```python
from build123d import *

# Parameters (mm, degrees)
F1_W     = 3
F1_H     = 5.5
F1_H_2   = 7.5
F1_H_3   = 5
F1_H_4   = 3
F1_W_2   = 17.5
F1_W_3   = 10
F2_DEPTH = 3
F3_DEPTH = 20
F0_W     = 5
F0_H     = 5
F0_R     = 1.5
F4_DEPTH = 11
F5_DEPTH = 15
F6_R     = 2
F1_H_5   = 59
F7_DEPTH = 1


with BuildPart() as f2:
    # F1 (on Top) → F2 (new body)
    with BuildSketch(Plane.XY):
        with Locations((-6.5, -41.25)):
            Rectangle(F1_W, F1_H)
        with Locations((-6.5, 40.25)):
            Rectangle(F1_W, F1_H_2)
        with Locations((-6.5, 34)):
            Rectangle(F1_W, F1_H_3)
        with Locations((-6.5, 30)):
            Rectangle(F1_W, F1_H_4)
        with Locations((-6.5, -36)):
            Rectangle(F1_W, F1_H_3)
        with Locations((-6.5, -32)):
            Rectangle(F1_W, F1_H_4)
        Polygon((43, -47), (43, -44), (25.5, -44), (8, -44), (5, -44), (-5, -44), (-8, -44), (-25.5, -44), (-43, -44), (-43, -47), align=None)
        Polygon((43, -38.5), (43, -44), (43, -47), (46, -47), (46, 47), (-46, 47), (-46, -47), (-43, -47), (-43, -44), (-43, -38.5), (-43, -33.5), (-43, -30.5), (-43, 28.5), (-43, 31.5), (-43, 36.5), (-43, 44), (-25.5, 44), (-8, 44), (-5, 44), (5, 44), (8, 44), (25.5, 44), (43, 44), (43, 36.5), (43, 31.5), (43, 28.5), (43, -30.5), (43, -33.5), align=None)
        with Locations((-34.25, 40.25)):
            Rectangle(F1_W_2, F1_H_2)
        with Locations((0, 40.25)):
            Rectangle(F1_W_3, F1_H_2)
        with Locations((6.5, 40.25)):
            Rectangle(F1_W, F1_H_2)
        with Locations((34.25, 40.25)):
            Rectangle(F1_W_2, F1_H_2)
        with Locations((34.25, 34)):
            Rectangle(F1_W_2, F1_H_3)
        with Locations((6.5, 34)):
            Rectangle(F1_W, F1_H_3)
        with Locations((-34.25, 34)):
            Rectangle(F1_W_2, F1_H_3)
        with Locations((0, 34)):
            Rectangle(F1_W_3, F1_H_3)
        with Locations((-34.25, 30)):
            Rectangle(F1_W_2, F1_H_4)
        with Locations((6.5, 30)):
            Rectangle(F1_W, F1_H_4)
        with Locations((34.25, 30)):
            Rectangle(F1_W_2, F1_H_4)
        with Locations((0, 30)):
            Rectangle(F1_W_3, F1_H_4)
        with Locations((0, -41.25)):
            Rectangle(F1_W_3, F1_H)
        with Locations((0, -36)):
            Rectangle(F1_W_3, F1_H_3)
        with Locations((0, -32)):
            Rectangle(F1_W_3, F1_H_4)
        with Locations((6.5, -41.25)):
            Rectangle(F1_W, F1_H)
        with Locations((6.5, -36)):
            Rectangle(F1_W, F1_H_3)
        with Locations((6.5, -32)):
            Rectangle(F1_W, F1_H_4)
        with Locations((-34.25, -32)):
            Rectangle(F1_W_2, F1_H_4)
        with Locations((34.25, -32)):
            Rectangle(F1_W_2, F1_H_4)
        with Locations((34.25, -36)):
            Rectangle(F1_W_2, F1_H_3)
        with Locations((-34.25, -36)):
            Rectangle(F1_W_2, F1_H_3)
        with Locations((-34.25, -41.25)):
            Rectangle(F1_W_2, F1_H)
        with Locations((34.25, -41.25)):
            Rectangle(F1_W_2, F1_H)
    extrude(amount=F2_DEPTH)

    # F1 (on Top) → F3 (join)
    with BuildSketch(Plane.XY):
        Polygon((43, -38.5), (43, -44), (43, -47), (46, -47), (46, 47), (-46, 47), (-46, -47), (-43, -47), (-43, -44), (-43, -38.5), (-43, -33.5), (-43, -30.5), (-43, 28.5), (-43, 31.5), (-43, 36.5), (-43, 44), (-25.5, 44), (-8, 44), (-5, 44), (5, 44), (8, 44), (25.5, 44), (43, 44), (43, 36.5), (43, 31.5), (43, 28.5), (43, -30.5), (43, -33.5), align=None)
    extrude(amount=F3_DEPTH)

    # F0 (on Top) → F4 (join)
    with BuildSketch(Plane.XY):
        with Locations((37.5, 34)):
            Rectangle(F0_W, F0_H)
        with Locations((37.5, 34)):
            Circle(F0_R, mode=Mode.SUBTRACT)
        with Locations((2.5, 34)):
            Rectangle(F0_W, F0_H)
        with Locations((2.5, 34)):
            Circle(F0_R, mode=Mode.SUBTRACT)
        with Locations((-2.5, 34)):
            Rectangle(F0_W, F0_H)
        with Locations((-2.5, 34)):
            Circle(F0_R, mode=Mode.SUBTRACT)
        with Locations((-37.5, 34)):
            Rectangle(F0_W, F0_H)
        with Locations((-37.5, 34)):
            Circle(F0_R, mode=Mode.SUBTRACT)
        with Locations((37.5, -36)):
            Rectangle(F0_W, F0_H)
        with Locations((37.5, -36)):
            Circle(F0_R, mode=Mode.SUBTRACT)
        with Locations((-2.5, -36)):
            Rectangle(F0_W, F0_H)
        with Locations((-2.5, -36)):
            Circle(F0_R, mode=Mode.SUBTRACT)
        with Locations((2.5, -36)):
            Rectangle(F0_W, F0_H)
        with Locations((2.5, -36)):
            Circle(F0_R, mode=Mode.SUBTRACT)
        with Locations((-37.5, -36)):
            Rectangle(F0_W, F0_H)
        with Locations((-37.5, -36)):
            Circle(F0_R, mode=Mode.SUBTRACT)
        with Locations((37.5, 34)):
            Circle(F0_R)
        with Locations((2.5, 34)):
            Circle(F0_R)
        with Locations((-2.5, 34)):
            Circle(F0_R)
        with Locations((-37.5, 34)):
            Circle(F0_R)
        with Locations((37.5, -36)):
            Circle(F0_R)
        with Locations((-2.5, -36)):
            Circle(F0_R)
        with Locations((2.5, -36)):
            Circle(F0_R)
        with Locations((-37.5, -36)):
            Circle(F0_R)
    extrude(amount=F4_DEPTH)

    # F0 (on Top) → F5 (join)
    with BuildSketch(Plane.XY):
        with Locations((37.5, -36)):
            Circle(F0_R)
        with Locations((2.5, -36)):
            Circle(F0_R)
        with Locations((-2.5, -36)):
            Circle(F0_R)
        with Locations((-37.5, -36)):
            Circle(F0_R)
        with Locations((-37.5, 34)):
            Circle(F0_R)
        with Locations((-2.5, 34)):
            Circle(F0_R)
        with Locations((2.5, 34)):
            Circle(F0_R)
        with Locations((37.5, 34)):
            Circle(F0_R)
    extrude(amount=F5_DEPTH)

    # F6
    f6_edges = [f2.edges().sort_by_distance(p)[0] for p in [
        (-37.5, -38.5, 3),
        (-35, -36, 3),
        (-37.5, -33.5, 3),
        (-40, -36, 3),
        (0, -38.5, 3),
        (-37.5, 31.5, 3),
        (0, 31.5, 3),
        (37.5, -38.5, 3),
        (5, -36, 3),
        (5, 34, 3),
        (-35, 34, 3),
        (-5, 34, 3),
        (-5, -36, 3),
        (35, 34, 3),
        (37.5, 31.5, 3),
        (35, -36, 3),
        (0, -33.5, 3),
        (40, -36, 3),
        (37.5, -33.5, 3),
        (-37.5, 36.5, 3),
        (-40, 34, 3),
        (0, 36.5, 3),
        (37.5, 36.5, 3),
        (40, 34, 3),
    ]]
    fillet(f6_edges, radius=F6_R)

    # F1 (on Top) → F7 (join)
    with BuildSketch(Plane.XY):
        with Locations((0, -1)):
            Rectangle(F1_W_3, F1_H_5)
    extrude(amount=F7_DEPTH)


solid = f2.part
```
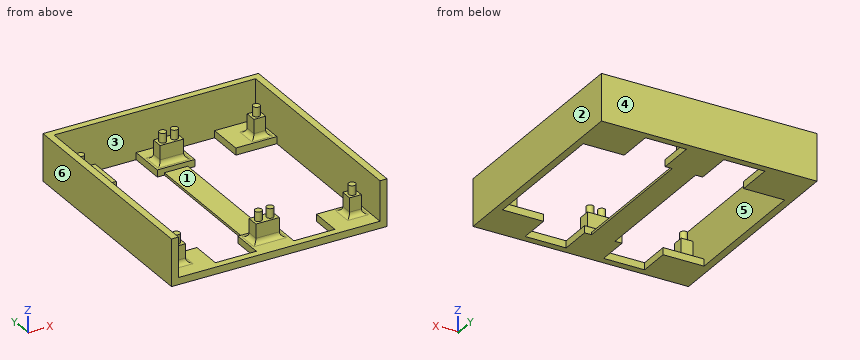
For this review, take the finished solid that the model builds, in its own axes (mm). Face numbers are marked on the shaded views. A direction names the side the tool comes from. Coordinates: 2 decimals unless noted, no trailing zeros. Order: outer loops, then holes, each group sorted by start corner. A loop starts at its lowest first (then second) coordinate and runs counter-clockwise, first axis right, second up. Notation, with made-up numbers: (-18, 1.5) - (30, 1.5) arc R23 ccw to (30, 15.5) - close; hole circle Ø5 at (58.5, 45). An arc over 180 degrees is marked (long way). Answer as a JSON object with one key per item and string values. Group by question number.
1. Clearance check with flat-ended pins moving along their axes: P1, Ø0.9, axis at x = 2.5, y = -36, coming from the +Z side; P2, Ø4, axis at x = 2.5, z = 12, coming from the -Y side; P3, Ø6, axis at x = 17, z = 12, coming from the -Y side. State where each tip first meets the part, or that it passes through.
2. We need section B-B on y = 13. State the section outline as (x, z) points, then the cut area to 3 significant figures.
3. The part is to be moulded in two halves that separate along X. For the marked faces 3, 4, 5 and 6, say which applies: pulls with the +X half, pulls with the -X half, needs draft (parallel to the pull), parting line crosses it, or undercut.
4. For the marked faces 1 and 2, list the 3-axis set-ups (+Z, -Z, +X, -X, +Y, -Y) from which the entire face can be reached by the end or side of a thin tool; tool diameter is ignored.
5. We need section A-A on x = -19. State the section outline as (y, z) points, then the cut area to 3 significant figures.
6. For probe 1 along Y at (x, z) = (4, 7.25); probe 2 along X at (y, z) = (-38, 8.5); probe 3 along X at (y, z) = (16, 5.75), list the stretches that pass through material, from the lowest coordinate up.
Final values:
{
 "1": {"P1": "z = 15", "P2": "y = -38.5", "P3": "y = 44"},
 "2": {"outline": "(-46, 0) - (-43, 0) - (-43, 20) - (-46, 20) - close; (-5, 0) - (5, 0) - (5, 1) - (-5, 1) - close; (43, 0) - (46, 0) - (46, 20) - (43, 20) - close", "area": "130 mm²"},
 "3": {"face 3": "undercut", "face 4": "needs draft", "face 5": "undercut", "face 6": "pulls with the -X half"},
 "4": {"face 1": "+Z", "face 2": "+Z, -Z, +X, +Y, -Y"},
 "5": {"outline": "(-47, 0) - (-44, 0) - (-44, 3) - (-47, 3) - close; (44, 0) - (47, 0) - (47, 20) - (44, 20) - close", "area": "69.0 mm²"},
 "6": {"probe 1": "-38.5 to -33.5, 31.5 to 36.5, 44 to 47", "probe 2": "-46 to -43, -40 to -35, -5 to 5, 35 to 40, 43 to 46", "probe 3": "-46 to -43, 43 to 46"}
}
